from build123d import *

# Parameters (mm, degrees)
F0_W      = 10
F0_H      = 30
F0_W_2    = 5
F0_W_3    = 30
F0_H_2    = 10
F0_W_4    = 25
F0_H_3    = 15
F1_DEPTH  = 4
F2_W      = 16
F2_H      = 16
F2_H_2    = 4
F3_DEPTH  = 4
F5_D      = 8.1
F7_DEPTH  = 3
F8_W      = 80
F8_H      = 10.0841035172
F8_H_2    = 4
F9_DEPTH  = 4
F11_D     = 3.1
F12_R     = 1.45
F13_DEPTH = 3
F14_R     = 1.45
F15_DEPTH = 4
F17_D     = 3.1


with BuildPart() as f1:
    # F0 (on Top) → F1 (new body)
    with BuildSketch(Plane.XY):
        with Locations((-48, 67)):
            Rectangle(F0_W, F0_H)
        Polygon((-10, 42), (-10, 52), (-43, 52), (-53, 52), (-53, 42), align=None)
        with Locations((-2.5, 67)):
            Rectangle(F0_W_2, F0_H)
        with Locations((2.5, 67)):
            Rectangle(F0_W_2, F0_H)
        Polygon((-5, 52), (-10, 52), (-10, 42), (-10, -42), (-10, -52), (10, -52), (10, -42), (10, 42), (10, 52), (5, 52), (0, 52), align=None)
        with Locations((-25, -47)):
            Rectangle(F0_W_3, F0_H_2)
        with Locations((25, -47)):
            Rectangle(F0_W_3, F0_H_2)
        with Locations((40.5, 34.5)):
            Rectangle(F0_W_4, F0_H_3)
        Polygon((43, 52), (10, 52), (10, 42), (28, 42), (53, 42), (53, 52), align=None)
        with Locations((48, 67)):
            Rectangle(F0_W, F0_H)
    extrude(amount=F1_DEPTH)

    # F2 (on face) → F3 (join)
    with BuildSketch(Plane.XZ.offset(-42)):
        with Locations((-45, 12)):
            Rectangle(F2_W, F2_H)
        with Locations((-45, 2)):
            Rectangle(F2_W, F2_H_2)
    extrude(amount=F3_DEPTH)

    # F5 (through all)
    with Locations(Plane.XZ.offset(-38)):
        with Locations((-45, 12.6515012234)):
            Hole(F5_D / 2)

    # F6 (on face) → F7 (join)
    with BuildSketch(Plane(origin=(-53, 0, 0), x_dir=(0, -1, 0), z_dir=(-1, 0, 0))):
        Polygon((-42, 20), (-45.4689958334, 4), (-42, 4), align=None)
        Polygon((-45.4689958334, 4), (-46.3362447917, 0), (-38, 0), (-38, 20), (-42, 20), (-42, 4), align=None)
    extrude(amount=F7_DEPTH)

    # F8 (on face) → F9 (join)
    with BuildSketch(Plane.XZ.offset(52)):
        with Locations((0, 9.0420517586)):
            Rectangle(F8_W, F8_H)
        with Locations((0, 2)):
            Rectangle(F8_W, F8_H_2)
    extrude(amount=F9_DEPTH)

    # F11 (through all)
    with Locations(Plane.XY.offset(4)):
        with Locations((-20, 46.8481220305), (20, 46.8481220305), (-48, 77.2035785913), (0, 77.2035785913), (71.8699040711, 77.2035785913)):
            Hole(F11_D / 2)

    # F12 (on face) → F13 (join)
    with BuildSketch(Plane.XY.offset(4)):
        with Locations((0, -43)):
            Circle(F12_R)
    extrude(amount=F13_DEPTH)

    # F14 (on face) → F15 (join)
    with BuildSketch(Plane.XY.offset(7)):
        with BuildLine():
            ThreePointArc((-3.4964729281, -41.0571471845), (-1.0035208736, -46.8720725531), (4, -43))
            ThreePointArc((4, -43), (3.8720725531, -41.9964791264), (3.4964729281, -41.0571471845))
            Line((3.4964729281, -41.0571471845), (-3.4964729281, -41.0571471845))
        make_face()
        with Locations((0, -43)):
            Circle(F14_R, mode=Mode.SUBTRACT)
        with Locations((0, -43)):
            Circle(F14_R)
    extrude(amount=F15_DEPTH)

    # F17 (through all)
    with Locations(Plane.XY.offset(4)):
        with Locations((47.9784347117, 77.9637917876)):
            Hole(F17_D / 2)


solid = f1.part
Geometry check sheet. Reference: the model listing, model coordinates, mm. A direction names the side the tool comes from. Give positions to 0.01 mm unless a question says otherwise; leave off trailing zeros. Write each loop counter-clockwise with the first axis right and the second up, starting at its lowest first coordinate (ties: lowest second). Pieces come first, ordered by that corner, then holes.
1) Cross-section at D-D (x = 0). Record the boundary of the cut face in (y, z).
Values follow:
outline: (-56, 0) - (75.65, 0) - (75.65, 4) - (-41.55, 4) - (-41.55, 7) - (-41.06, 7) - (-41.06, 11) - (-47, 11) - (-47, 7) - (-44.45, 7) - (-44.45, 4) - (-52, 4) - (-52, 14.08) - (-56, 14.08) - close; (78.75, 0) - (82, 0) - (82, 4) - (78.75, 4) - close
2) Cross-section at A-A (y = 28.5). Record the boundary of the cut face in (x, z), plus the area to 3 significant figures.
Values follow:
outline: (-10, 0) - (10, 0) - (10, 4) - (-10, 4) - close; (28, 0) - (53, 0) - (53, 4) - (28, 4) - close
area: 180 mm2
3) Set-up check for faces 4 (the face through (43, 67, 2)), 5 (the face through (0, -41.057, 9)), 6 (the face through (-25, -42, 2)), 7 (the face through (19, 42, 2)): record each of +Z, -Z, +X, -X, +Y, -Y from which the full face is reachable in a straight line by a thin tool's end or side.
Values follow:
face 4: +Z, -Z, +Y
face 5: +Z, +X, -X, +Y
face 6: +Z, -Z, -X
face 7: +Z, -Z
4) Cross-section at C-C (y = 69). Record the boundary of the cut face in (x, z).
Values follow:
outline: (-53, 0) - (-43, 0) - (-43, 4) - (-53, 4) - close; (-5, 0) - (5, 0) - (5, 4) - (-5, 4) - close; (43, 0) - (53, 0) - (53, 4) - (43, 4) - close
5) Thickness scan on line 1 (X direction, y = 75.5, z = 3.5); line 2 (Y direction, x = 20, z = 2.8); line 3 (Y direction, x = -48, z = 1.05). Record the ranges inside material, lowest first.
Values follow:
line 1: x = -53 to -43, -5 to 5, 43 to 53
line 2: y = -56 to -42, 42 to 45.3, 48.4 to 52
line 3: y = 38 to 75.65, 78.75 to 82
6) Go/stop test with flat-tipped pins: pin 1 Ø2 at (y, z) = (35.5, 2.5) entering from -X; pin 2 Ø7 at (y, z) = (-50.5, 9) entering from -X; pin 3 Ø4 at (x, y) = (-41, 51) entering from -Z; pin 4 Ø4.5 at (x, y) = (-18, -53) entering from +Z. Record where each tip stops, or that it passes through.
Values follow:
pin 1: stops at x = -10
pin 2: stops at x = -40
pin 3: stops at z = 0
pin 4: stops at z = 14.08
7) Cross-section at B-B (x = -20). Record the boundary of the cut face in (y, z).
Values follow:
outline: (-56, 0) - (-42, 0) - (-42, 4) - (-52, 4) - (-52, 14.08) - (-56, 14.08) - close; (42, 0) - (45.3, 0) - (45.3, 4) - (42, 4) - close; (48.4, 0) - (52, 0) - (52, 4) - (48.4, 4) - close
8) Release check for a two-part mould opening along X. For faces 1 (the face through (-5, 67, 2)), 2 (the face through (-53, 43, 9)), 3 (the face through (40, 27, 2)) record: released by +X, released by -X, zero draft, split by the parting line, or undercut.
Values follow:
face 1: undercut
face 2: released by +X
face 3: zero draft
